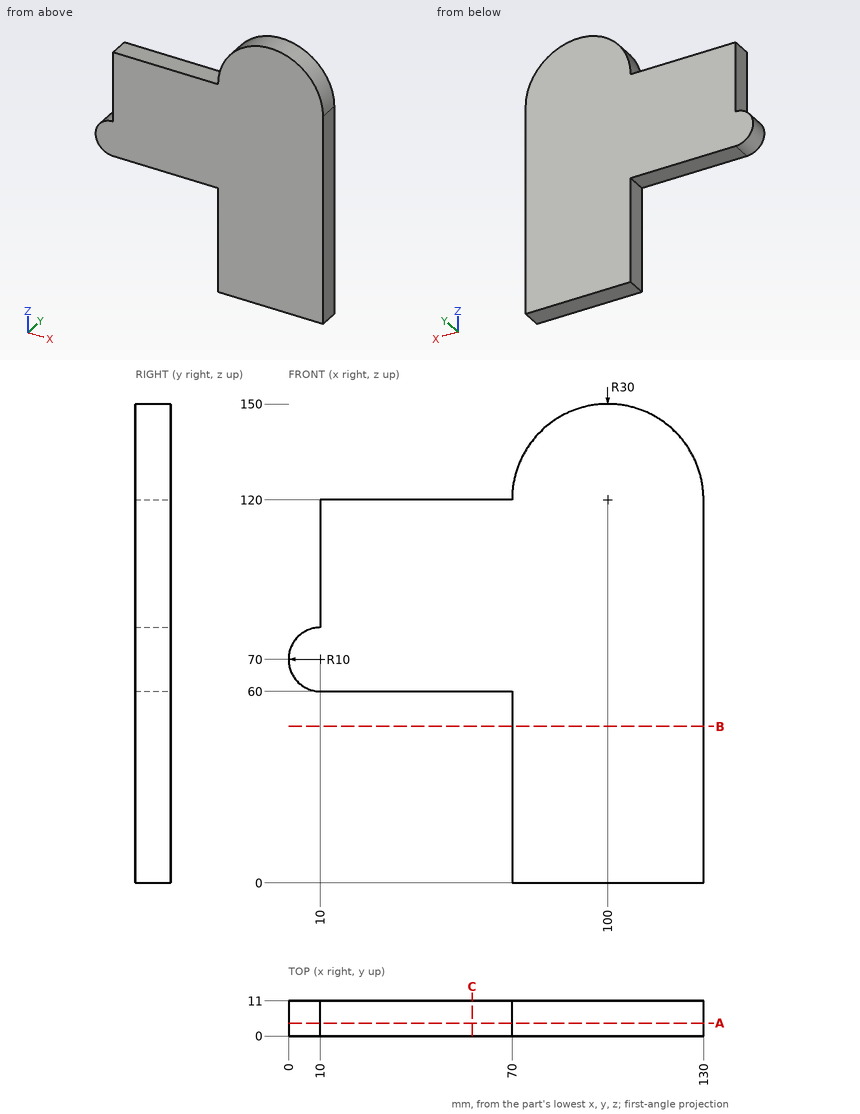
Geometry: see drawing. Coordinates: mm, zero at the bounding-box minimum. Round coordinates to 2 decimals unless told otherwise and drop trailing zeros. Loops run counter-clockwise (first coordinate to the right, second up) from the corner with the lowest first, then second, coordinate; pieces in that order, holes last. Notation, with made-up numbers: M 51,-19 L 88,-19 A16 ccw 88,-6 Z; hole C -15,-3.5 d11. An arc over 180 degrees is marked long. Use a Markdown table: item, result. Add a question column.
1. Section query A-A on y = 4. Return the cut outline in (x, z), then the cut area to 3 significant figures.
2. Contact query for flat-ended pins moving along their axis: P1, Ø5.5, axis at y = 3.5, z = 31.5, coming from the -X side; P2, Ø1.5, axis at x = 54.5, z = 102.5, coming from the -Y side; P3, Ø5.5, axis at x = 35, y = 6.5, coming from the -Z side; P4, Ø3.5, axis at y = 6.5, z = 100.5, coming from the -X side. Output: stop coordinate, or through.
3. Section query B-B on z = 49. Return the cut outline in (x, y), then the cut area to 3 significant figures.
4. Line query: line 1 (X direction, y = 9, z = 43.5); line 2 (Z direction, x = 15.5, y = 2); line 3 (X direction, y = 5, z = 97). Output: solid intervals per line, ascending.
5. Section query C-C on x = 57.5. Return the cut outline in (y, z).
Reported:
| question | item | result |
|---|---|---|
| 1 | outline | M 10,60 L 70,60 L 70,0 L 130,0 L 130,120 A30 ccw 70,120 L 10,120 L 10,80 A10 ccw Z |
| 1 | area | 12,400 mm² |
| 2 | P1 | stops at x = 70 |
| 2 | P2 | stops at y = 0 |
| 2 | P3 | stops at z = 60 |
| 2 | P4 | stops at x = 10 |
| 3 | outline | M 70,0 L 130,0 L 130,11 L 70,11 Z |
| 3 | area | 660 mm² |
| 4 | line 1 | x = 70 to 130 |
| 4 | line 2 | z = 60 to 120 |
| 4 | line 3 | x = 10 to 130 |
| 5 | outline | M 0,60 L 11,60 L 11,120 L 0,120 Z |
